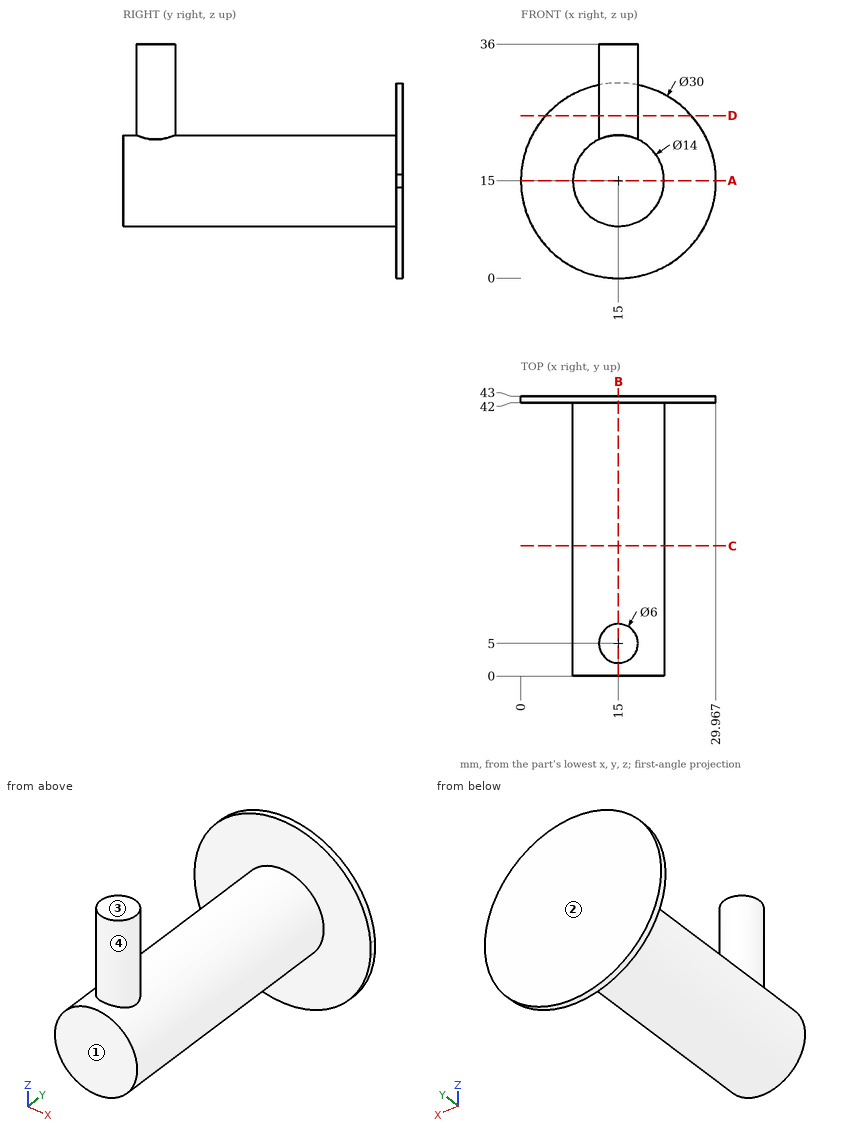
Study the drawing (mm; zero at the part's minimum x, y, z) and answer. Give positions to 0.01 mm unless a question says otherwise; leave off trailing zeros. Order: outer loops, then holes, each group sorted by start corner. A loop starts at its lowest first (then second) coordinate and runs counter-clockwise, first axis right, second up. Notation, with made-up numbers: (88, -24) - (115, -24) arc R18 ccw to (115, 9) - close; hole circle Ø5 at (-27, 82.5). An arc over 180 degrees is marked (long way). Answer in a Markdown table with one row per item. Add a question column.
Q1. Find the intervals of material crossed by line 1 along Y through (x, z) = (21.5, 28); line 2 along Y through (x, z) = (13.75, 28.5); line 3 along X through (y, z) = (10, 17), in increasing order. Write a range as [from, to].
Q2. The part is cut by section C-C (y = 20). Determine the outline of the cut face in (x, z), then the cut area to 3 significant figures.
Q3. The part is cut by section A-A (z = 15). Determine the outline of the cut face in (x, y).
Q4. Given P1, Ø5, axis at x = 11.5, y = 22.5, coming from the -Z side; P2, Ø10, axis at x = 19.5, y = 38, coming from the +Z side (1 decimal); P3, Ø1.5, axis at y = 6, z = 30.5, coming from the +X side, each flat-ended and moving along its own axis, determine where each tip first touches the part or whether it passes through.
Q5. For a pull along Y with two mould halves and no side action, classify the marked faces 1, 2, 3 and 4 as released by +Y, released by -Y, zero draft, split by the parting line, or undercut.
Q6. The part is cut by section D-D (z = 25). Determine the outline of the cut face in (x, y).
Q7. The part is cut by section B-B (x = 15). Determine the outline of the cut face in (y, z).
Determined:
| question | item | result |
|---|---|---|
| 1 | line 1 | y = [42, 43] |
| 1 | line 2 | y = [2.27, 7.73], [42, 43] |
| 1 | line 3 | x = [8.29, 21.71] |
| 2 | outline | circle Ø14 at (15, 15) |
| 2 | area | 154 mm² |
| 3 | outline | (0, 42) - (8, 42) - (8, 0) - (22, 0) - (22, 42) - (29.97, 42) - (29.97, 43) - (0, 43) - close |
| 4 | P1 | stops at z = 8.07 |
| 4 | P2 | stops at z = 29.9 |
| 4 | P3 | stops at x = 17.99 |
| 5 | face 1 | released by -Y |
| 5 | face 2 | released by +Y |
| 5 | face 3 | zero draft |
| 5 | face 4 | undercut |
| 6 | outline | (3.82, 42) - (26.18, 42) - (26.18, 43) - (3.82, 43) - close; circle Ø6 at (15, 5) |
| 7 | outline | (0, 8) - (42, 8) - (42, 0) - (43, 0) - (43, 30) - (42, 30) - (42, 22) - (8, 22) - (8, 36) - (2, 36) - (2, 22) - (0, 22) - close |
